Source: three-view drawing plus pictorial views. Frame: mm from the lowest corner of the part. Round coordinates to 2 decimals unless told otherwise and drop trailing zeros. Loops run counter-clockwise (first coordinate to the right, second up) from the corner with the lowest first, then second, coordinate; pieces in that order, holes last. Notation, with made-up numbers: (-32, 71.5) -> (-6, 71.5) arc R30 cw to (-6, 107.5) -> close; hole circle Ø8 at (51, 76.25). An arc over 180 degrees is marked (long way). One line per question, with ' | ' between items. Start each with the question number.
Q1. Cut plane B-B on x = 603.5. Return loops of the section in (y, z).
Q2. Contact query for flat-ended pins moving along their axis: P1, Ø1.5, axis at y = 7, z = 89, coming from the -X side; P2, Ø1, axis at y = 3, z = 70.5, coming from the +X side. Output: stop coordinate, or through.
Q3. Material intervals for L1, parallel to Z at x = 547.5, y = 7.75; L2, parallel to Z at x = 511, y = 4.25; L3, parallel to X at y = 5, z = 82, sorted ascending.
Q4. Cut plane A-A on z = 29. Return loops of the section in (x, y), and give its area (3 significant figures).
Q5. Cut plane C-C on y = 5. Return loops of the section in (x, z), and give its area (3 significant figures).
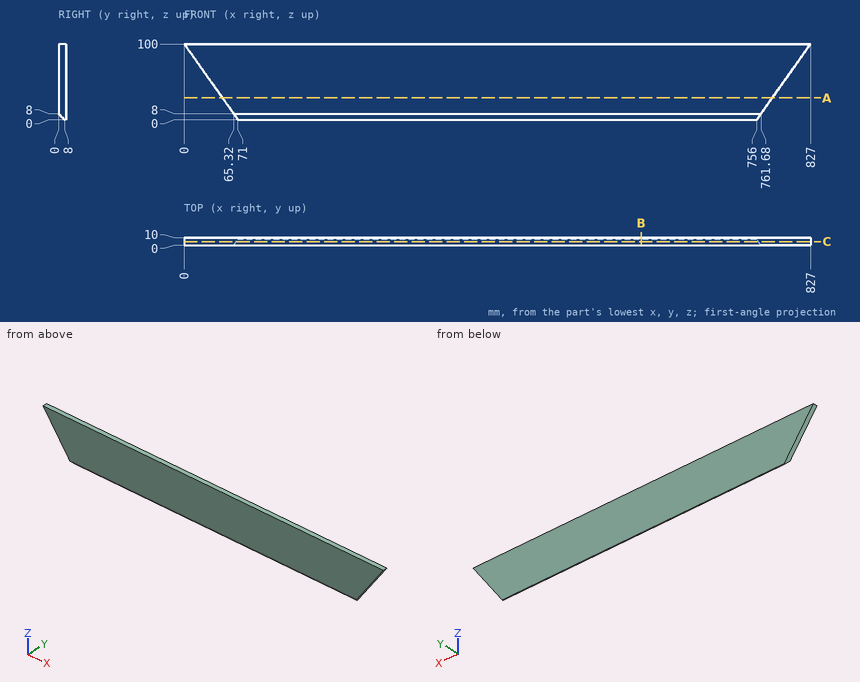
Results:
1) outline: (0, 8) -> (8, 0) -> (10, 0) -> (10, 100) -> (0, 100) -> close
2) P1: x = 7.28 | P2: x = 806.41
3) L1: 0.25 to 100 | L2: 3.75 to 100 | L3: 12.78 to 814.22
4) outline: (50.41, 0) -> (776.59, 0) -> (776.59, 10) -> (50.41, 10) -> close | area: 7,260 mm^2
5) outline: (0, 100) -> (68.87, 3) -> (758.13, 3) -> (827, 100) -> close | area: 73,500 mm^2
